Autodesk Inventor part; units mm, degrees
ref_plane "YZ Plane" through (0, 0, 0) normal (1, 0, 0) x (0, 1, 0)
ref_plane "XZ Plane" through (0, 0, 0) normal (0, 1, 0) x (-1, 0, 0)
ref_plane "XY Plane" through (0, 0, 0) normal (0, 0, 1) x (1, 0, 0)
sketch "Sketch1" plane through (0, 0, 0) normal (0, 0, 1) x (1, 0, 0)
  circle A0 centre (0, 0) radius 13.92
  circle A1 centre (0, 0) radius 14.92
  line L0 (-10, -11.0728) -> (-15, -28)
  line L1 (-15, -28) -> (15, -28)
  line L2 (15, -28) -> (10, -11.0728)
  line L3 (8.3051, -12.3948) -> (12.0284, -25)
  line L4 (12.0284, -25) -> (-12.0284, -25)
  line L5 (-12.0284, -25) -> (-8.3051, -12.3948)
  line L6 (-2, -22) -> (2, -22) construction
  line L7 (2, -22) -> (2, -25) construction
  line L8 (2, -25) -> (-2, -25) construction
  line L9 (-2, -25) -> (-2, -22) construction
  line L10 (2.15, -21.7) -> (-2.15, -21.7)
  line L11 (-2.15, -21.7) -> (-2.15, -25)
  line L12 (-2.15, -25) -> (2.15, -25) construction
  line L13 (2.15, -25) -> (2.15, -25)
  line L14 (2.15, -25) -> (2.15, -21.7)
  line L15 (-2.15, -25) -> (-2.15, -25)
  line L16 (-3.15, -25) -> (-3.15, -20.7)
  line L17 (-3.15, -20.7) -> (3.15, -20.7)
  line L18 (3.15, -20.7) -> (3.15, -25)
  line L19 (-1.48, 13.8411) -> (-1.48, 10.8811) construction
  line L20 (-1.48, 10.8811) -> (1.48, 10.8811) construction
  line L21 (1.48, 10.8811) -> (1.48, 13.8411) construction
  line L22 (1.33, 13.8563) -> (1.33, 11.0311)
  line L23 (1.33, 11.0311) -> (-1.33, 11.0311)
  line L24 (-1.33, 11.0311) -> (-1.33, 13.8563)
  line L25 (-1.33, -13.8563) -> (-1.33, -11.0311)
  line L26 (-1.33, -11.0311) -> (1.33, -11.0311)
  line L27 (1.33, -11.0311) -> (1.33, -13.8563)
  line L28 (2, 20) -> (-2, 20) construction
  line L29 (-2, 20) -> (-2, 17) construction
  line L30 (-2, 17) -> (2, 17) construction
  line L31 (2, 17) -> (2, 20) construction
  line L32 (-2.15, 16.85) -> (-2.15, 20.15)
  line L33 (-2.15, 20.15) -> (2.15, 20.15)
  line L34 (2.15, 20.15) -> (2.15, 16.85)
  line L35 (2.15, 16.85) -> (-2.15, 16.85)
  line L36 (3.15, 14.5837) -> (3.15, 21.15)
  line L37 (3.15, 21.15) -> (-3.15, 21.15)
  line L38 (-3.15, 21.15) -> (-3.15, 14.5837)
  point P0 (0, -22)
  point P1 (0, 10.8811)
  point P2 (0, 20)
  dimension "d0" = 27.84
  dimension "d1" = 1
  dimension "d2" = 3
  dimension "d3" = 2
  dimension "d4" = 2
  dimension "d5" = 28
  dimension "d6" = 30
  dimension "d7" = 20
  dimension "d10" = 3
  dimension "d11" = 4
  dimension "d12" = 3
  dimension "d13" = 0.3
  dimension "d14" = 0.15
  dimension "d15" = 0.15
  dimension "d16" = 1
  dimension "d17" = 1
  dimension "d18" = 1
  dimension "d22" = 2.96
  dimension "d23" = 2.96
  dimension "d24" = 0.15
  dimension "d25" = 0.15
  dimension "d26" = 0.15
  dimension "d30" = 3
  dimension "d31" = 4
  dimension "d32" = 17
  dimension "d33" = 0.15
  dimension "d34" = 1
  dimension "d35" = 1
  dimension "d36" = 1
extrude "Extrusion1" add sketch "Sketch1" along normal blind 10 contours A1 | A1 L38 L37 L36 | L2 L1 L0 A1 L5 L4 L3 | L4 L14 L10 L11 L16 L17 L18
fillet "Fillet1" radius 4 6 edges at (10, -11.0728, 5) (-10, -11.0728, 5) (-8.3051, -12.3948, 5) (8.3051, -12.3948, 5) (3.15, 14.5837, 5) (-3.15, 14.5837, 5)
fillet "Fillet1" radius 2 4 edges at (-12.0284, -25, 5) (12.0284, -25, 5) (3.15, -25, 5) (-3.15, -25, 5)
fillet "Fillet1" radius 1 4 edges at (-3.15, -20.7, 5) (3.15, -20.7, 5) (3.15, 21.15, 5) (-3.15, 21.15, 5)
extrude "Extrusion2" add sketch "Sketch1" along normal blind 4.3 contours L22 L23 L24 A0 | A0 L25 L26 L27
fillet "Fillet2" radius 2 2 edges at (0, -11.0311, 4.3) (0, 11.0311, 4.3)
properties part number "Motor Reversed Mount" material "ABS Plastic"
Geometry: final body of the model. Coordinates: model frame, mm. A direction names the side the tool comes from. Round coordinates to 2 decimals unless told otherwise and drop trailing zeros. Order: outer loops, then holes, each group sorted by start corner. A loop starts at its lowest first (then second) coordinate and runs counter-clockwise, first axis right, second up.
Q1. Section B-B, the plane y = 0. Output: boundary loops of the cut face in (x, z), and give its area (3 significant figures).
Result sheet:
outline: (-14.92, 0) - (-13.92, 0) - (-13.92, 10) - (-14.92, 10) - close; (13.92, 0) - (14.92, 0) - (14.92, 10) - (13.92, 10) - close
area: 20.0 mm2
Q2. Section C-C, the plane x = 12.5. Output: boundary loops of the cut face in (y, z).
Result sheet:
outline: (-28, 0) - (-19.54, 0) - (-19.54, 10) - (-28, 10) - close; (-8.15, 0) - (-6.13, 0) - (-6.13, 10) - (-8.15, 10) - close; (6.13, 0) - (8.15, 0) - (8.15, 10) - (6.13, 10) - close
Q3. Section D-D, the plane y = 12. Output: boundary loops of the cut face in (x, z).
Result sheet:
outline: (-8.87, 0) - (-7.05, 0) - (-7.05, 10) - (-8.87, 10) - close; (-1.33, 0) - (1.33, 0) - (1.33, 4.01) - (-1.33, 4.01) - close; (7.05, 0) - (8.87, 0) - (8.87, 10) - (7.05, 10) - close
Q4. Mould query, pull axis X, two halves, no side actions, for faces 1 (the face through (0, -21.7, 5)), 2 (the face through (14.435, 3.774, 4.93)), 3 (the face through (-2.849, 20.865, 5.07)). Classes: released by +X, released by -X, zero draft, split by the parting line, or undercut.
Result sheet:
face 1: undercut
face 2: released by +X
face 3: released by -X
Q5. Material intervals for probe 1 along Y at (x, z) = (0.5, 6); probe 2 along X at (y, z) = (19, 6.75); probe 3 along Y at (x, z) = (0, 3.5), sorted ascending.
Result sheet:
probe 1: y = -28 to -25, -21.7 to -20.7, -14.91 to -13.91, 13.91 to 16.85, 20.15 to 21.15
probe 2: x = -3.15 to -2.15, 2.15 to 3.15
probe 3: y = -28 to -25, -21.7 to -20.7, -14.92 to -11.43, 11.43 to 16.85, 20.15 to 21.15
Q6. Pin query (flat end, axial travel): pin 1 (0.7 mm diameter, centred on x = 0, y = -13.5, fed in from +Z); pin 2 (2 mm diameter, centred on x = 7, y = 15, fed in from -Z); pin 3 (2.5 mm diameter, centred on y = 19, z = 7.5, fed in from +X); pin 4 (2 mm diameter, centred on x = -7, z = 5, fed in from +Y). Return the tip coordinate at first contact, or that it passes through.
Result sheet:
pin 1: stops at z = 4.3
pin 2: passes through
pin 3: stops at x = 3.15
pin 4: stops at y = 13.66
Q7. Access query for faces 4 (the face through (3.15, 19, 5)), 5 (the face through (10.583, -11.319, 5.07)), 6 (the face through (0, -12, 0)), 7 (the face through (2.15, -23, 5)), 8 (the face through (0.019, -11.601, 3.699)). Directions: +Z, -Z, +X, -X, +Y, -Y. A direction counts if a zero-diameter tool reaches every point of the face in a straight line with its end or side. Return the directions, or none.
Result sheet:
face 4: +Z, -Z, +X, +Y
face 5: +Z, -Z, +X
face 6: -Z, +X, -X, +Y, -Y
face 7: +Z, -Z
face 8: +Z
Q8. Section A-A, the plane x = 0. Output: boundary loops of the cut face in (y, z).
Result sheet:
outline: (-28, 0) - (-25, 0) - (-25, 10) - (-28, 10) - close; (-21.7, 0) - (-20.7, 0) - (-20.7, 10) - (-21.7, 10) - close; (-14.92, 0) - (-11.03, 0) - (-11.03, 2.3) arc R2 ccw to (-13.03, 4.3) - (-13.92, 4.3) - (-13.92, 10) - (-14.92, 10) - close; (11.03, 0) - (16.85, 0) - (16.85, 10) - (13.92, 10) - (13.92, 4.3) - (13.03, 4.3) arc R2 ccw to (11.03, 2.3) - close; (20.15, 0) - (21.15, 0) - (21.15, 10) - (20.15, 10) - close
